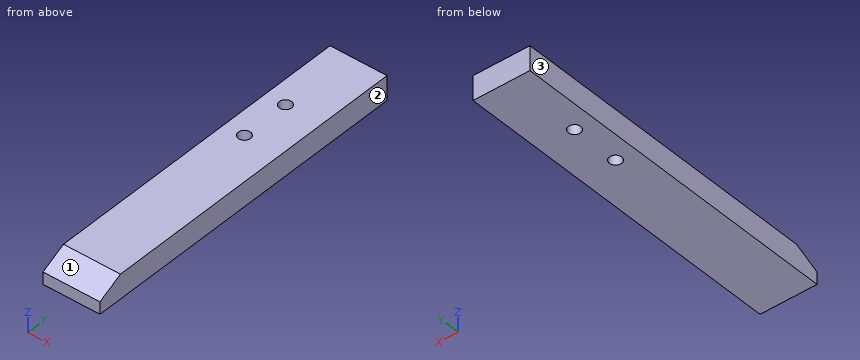
```python
from build123d import *

# Parameters (mm, degrees)
F0_W     = 88.9
F0_H     = 38.1
F1_DEPTH = 266.7
F3_DEPTH = 88.901
F4_R     = 9.525
F5_DEPTH = 38.101


with BuildPart() as f1:
    # F0 (on Front) → F1 (new body, symmetric)
    with BuildSketch(Plane.XZ):
        with Locations((2.043676, -0.6204)):
            Rectangle(F0_W, F0_H)
    extrude(amount=F1_DEPTH, both=True)

    # F2 (on face) → F3 (cut, through all)
    with BuildSketch(Plane.YZ.offset(46.493676)):
        Polygon((-266.7, -0.6204), (-228.6, 18.4296), (-266.7, 18.4296), align=None)
    extrude(amount=-F3_DEPTH, mode=Mode.SUBTRACT)

    # F4 (on face) → F5 (cut, through all)
    with BuildSketch(Plane.XY.offset(18.4296)):
        with Locations((-10.656324, 146.05)):
            Circle(F4_R)
        with Locations((-10.656324, 69.85)):
            Circle(F4_R)
    extrude(amount=-F5_DEPTH, mode=Mode.SUBTRACT)


solid = f1.part
```
Geometry check sheet. Reference: the model listing, model coordinates, mm. Face numbers are marked on the shaded views. Coordinates: 2 decimals unless noted, no trailing zeros. Write each loop counter-clockwise with the first axis right and the second up, starting at its lowest first coordinate (ties: lowest second). Pieces come first, ordered by that corner, then holes. Notation, with made-up numbers: M 35,53.25 L 55,53.25 A21 ccw 55,63.25 Z; hole C 15.25,31.5 d3. An arc over 180 degrees is marked long. One line per item, written item: value. Start each with the question number.
(1) Sectioned sample at A-A, the plane y = 146.05. Enter the section's corners in (x, z), and give its area (3 significant figures).
(2) Sectioned sample at B-B, the plane z = 11.5. Enter the section's corners in (x, y) (3 decimals).
(3) Sectioned sample at C-C, the plane x = 27.5. Enter the section's corners in (y, z), and give its area (3 significant figures).
(4) Scan lines: line 1 along Y through (x, z) = (-13, -10.5); line 2 along Y through (x, z) = (-16, -14.5); line 3 along X through (y, z) = (69, 7). Record each from-to range of solid material in increasing order. Write a range as [from, to].
(5) Release check for a two-part mould opening along X. For the marked faces 1, 2 and 3 record: released by +X, released by -X, zero draft, split by the parting line, or undercut.
Filled sheet:
1. outline: M -42.41,-19.67 L -20.18,-19.67 L -20.18,18.43 L -42.41,18.43 Z; M -1.13,-19.67 L 46.49,-19.67 L 46.49,18.43 L -1.13,18.43 Z
1. area: 2,660 mm²
2. outline: M -42.406,-242.459 L 46.494,-242.459 L 46.494,266.7 L -42.406,266.7 Z; hole C -10.656,69.85 d19.05; hole C -10.656,146.05 d19.05
3. outline: M -266.7,-19.67 L 266.7,-19.67 L 266.7,18.43 L -228.6,18.43 L -266.7,-0.62 Z
3. area: 20,000 mm²
4. line 1: [-266.7, 60.62], [79.08, 136.82], [155.28, 266.7]
4. line 2: [-266.7, 61.97], [77.73, 138.17], [153.93, 266.7]
4. line 3: [-42.41, -20.14], [-1.17, 46.49]
5. face 1: zero draft
5. face 2: released by +X
5. face 3: released by -X
